Autodesk Inventor part; units mm, degrees
ref_plane "YZ Plane" through (0, 0, 0) normal (1, 0, 0) x (0, 1, 0)
ref_plane "XZ Plane" through (0, 0, 0) normal (0, 1, 0) x (-1, 0, 0)
ref_plane "XY Plane" through (0, 0, 0) normal (0, 0, 1) x (1, 0, 0)
sketch "Sketch1" plane through (0, 0, 0) normal (0, 1, 0) x (-1, 0, 0)
  line L0 (-10, 25) -> (-10, 0)
  line L1 (10, 0) -> (10, 25)
  line L2 (10, 0) -> (-10, 0) construction
  line L3 (10, 30) -> (-10, 30) construction
  line L4 (10, 25) -> (-10, 25) construction
  line L5 (0, 25) -> (0, 0) construction
  line L6 (10, 20) -> (-10, 20) construction
  line L7 (10, 20) -> (0, 20) construction
  line L8 (0, 20) -> (-10, 20) construction
  line L9 (0, 20) -> (5, 20) construction
  line L10 (0, 20) -> (-5, 20) construction
  line L11 (10, 35) -> (10, 25)
  line L12 (-10, 35) -> (-10, 25)
  line L13 (10, 35) -> (-10, 35)
  line L14 (5, 35) -> (5, 30)
  line L15 (-5, 35) -> (-5, 30)
  line L16 (-10, -25) -> (-10, 0)
  line L17 (10, 0) -> (10, -25)
  line L18 (10, -30) -> (-10, -30) construction
  line L19 (10, -25) -> (-10, -25) construction
  line L20 (0, -25) -> (0, 0) construction
  line L21 (10, -20) -> (-10, -20) construction
  line L22 (10, -20) -> (0, -20) construction
  line L23 (0, -20) -> (-10, -20) construction
  line L24 (0, -20) -> (5, -20) construction
  line L25 (0, -20) -> (-5, -20) construction
  line L26 (10, -35) -> (10, -25)
  line L27 (-10, -35) -> (-10, -25)
  line L28 (10, -35) -> (-10, -35)
  line L29 (5, -35) -> (5, -30)
  line L30 (-5, -35) -> (-5, -30)
  dimension "d84" = 5
  dimension "d127" = 20
extrude "Extrusion1" add sketch "Sketch1" along normal blind 5
hole "Hole12" at (-5, 0, 30) at (5, 0, 30) at (-5, 0, -30) at (5, 0, -30) direction (0, 1, 0) diameter 3.4 end through all
hole "Hole13" at (0, 0, 20) at (-5, 0, -20) at (5, 0, -20) direction (0, 1, 0) diameter 1.567 end through all
properties part number "mount-base" material "Copper"
Build history of the part. All positions in model axes, mm. Round coordinates to 2 decimals unless told otherwise and drop trailing zeros. Write each loop counter-clockwise with the first axis right and the second up, starting at its lowest first coordinate (ties: lowest second). Pieces come first, ordered by that corner, then holes. Notation, with made-up numbers: (-35, -29) - (9, -29) arc R17 ccw to (9, -15) - close; hole circle Ø8 at (-36, -29). An arc over 180 degrees is marked (long way). Write each question's results on one line, items separated by ' | '. Start each with the question number.
Item 1: Saw through at D-D (y = 3.05). Write the cut outline in (x, z), and give its area (3 significant figures).
Item 2: Saw through at B-B (x = 5). Write the cut outline in (y, z).
Item 3: Drop a flat-ended pin along its axis: P1, Ø0.9, axis at x = 5, z = -20, coming from the +Y side. Give the stop position or say it passes through.
Item 4: Saw through at C-C (z = -30). Write the cut outline in (x, y).
Item 5: Wall check: L1, parallel to Z at x = -5, y = 2.45; L2, parallel to X at y = 1.55, z = -20; L3, parallel to X at y = 4, z = 30. Give the ranges that are in metal, low to high. Write a range as [from, to].
Item 6: Mould opens along X. For faces 1 (the face through (0, 2, -35)), 2 (the face through (0.48, 2.54, 20.62)), 3 (the face through (10, 2, 0)) say: pulls with the +X half, pulls with the -X half, needs draft (parallel to the pull), parting line crosses it, or undercut.
Item 7: Saw through at A-A (x = 0). Write the cut outline in (y, z).
Results are:
1) outline: (-10, -35) - (10, -35) - (10, 35) - (-10, 35) - close; hole circle Ø3.4 at (-5, -30); hole circle Ø3.4 at (-5, 30); hole circle Ø1.57 at (-5, -20); hole circle Ø1.57 at (0, 20); hole circle Ø3.4 at (5, -30); hole circle Ø3.4 at (5, 30); hole circle Ø1.57 at (5, -20) | area: 1,360 mm²
2) outline: (0, -35) - (5, -35) - (5, -31.7) - (0, -31.7) - close; (0, -28.3) - (5, -28.3) - (5, -20.78) - (0, -20.78) - close; (0, -19.22) - (5, -19.22) - (5, 28.3) - (0, 28.3) - close; (0, 31.7) - (5, 31.7) - (5, 35) - (0, 35) - close
3) P1: passes through
4) outline: (-10, 0) - (-6.7, 0) - (-6.7, 5) - (-10, 5) - close; (-3.3, 0) - (3.3, 0) - (3.3, 5) - (-3.3, 5) - close; (6.7, 0) - (10, 0) - (10, 5) - (6.7, 5) - close
5) L1: z = [-35, -31.7], [-28.3, -20.78], [-19.22, 28.3], [31.7, 35] | L2: x = [-10, -5.78], [-4.22, 4.22], [5.78, 10] | L3: x = [-10, -6.7], [-3.3, 3.3], [6.7, 10]
6) face 1: needs draft | face 2: undercut | face 3: pulls with the +X half
7) outline: (0, -35) - (5, -35) - (5, 19.22) - (0, 19.22) - close; (0, 20.78) - (5, 20.78) - (5, 35) - (0, 35) - close
